from build123d import *

# Parameters (mm, degrees)
BOSS_EXTRUDE1_DEPTH            = 17
F_3_3_3_3_DIAMETER_HOLE1_D     = 3.3
F_3_3_3_3_DIAMETER_HOLE1_DEPTH = 25
F_3_3_3_3_DIAMETER_HOLE1_TIP   = 0.991420021


with BuildPart() as part:
    # Sketch1 → Boss-Extrude1 (new body)
    with BuildSketch(Plane.XY):
        with BuildLine():
            Line((-15, -23.643180835), (-15, -38))
            Line((-15, -38), (15, -38))
            Line((15, -38), (15, -23.643180835))
            ThreePointArc((15, -23.643180835), (0, 28), (-15, -23.643180835))
        make_face()
    extrude(amount=BOSS_EXTRUDE1_DEPTH)

    # Ø3.3 (3.3) Diameter Hole1
    with Locations(Plane.XY.offset(17)):
        with Locations((-23, 0), (23, 0)):
            Hole(F_3_3_3_3_DIAMETER_HOLE1_D / 2, depth=F_3_3_3_3_DIAMETER_HOLE1_DEPTH)
            with Locations((0, 0, -(F_3_3_3_3_DIAMETER_HOLE1_DEPTH + F_3_3_3_3_DIAMETER_HOLE1_TIP / 2))):  # 118° drill point
                Cone(0, F_3_3_3_3_DIAMETER_HOLE1_D / 2, F_3_3_3_3_DIAMETER_HOLE1_TIP, mode=Mode.SUBTRACT)


solid = part.part
Part model, mm, in its own coordinate system. A direction names the side the tool comes from. Coordinates: 2 decimals unless noted, no trailing zeros. Write each loop counter-clockwise with the first axis right and the second up, starting at its lowest first coordinate (ties: lowest second). Pieces come first, ordered by that corner, then holes. Notation, with made-up numbers: M 40,40.25 L 79,40.25 A23 cw 79,66.25 Z; hole C 12,70 d7. An arc over 180 degrees is marked long. Return JSON: item names as keys, results as strings.
1. Flat gauge pins, fed straight in: pin 1 Ø1 at (y, z) = (2.5, 12) entering from +X; pin 2 Ø4 at (y, z) = (17.5, 14.5) entering from -X; pin 3 Ø2 at (y, z) = (19.5, 8) entering from +X. Where does each tip first touch, or does it go through?
Determined:
{"pin 1": "x = 27.93", "pin 2": "x = -23.32", "pin 3": "x = 21.02"}
2. Saw through at D-D, the plane y = -28.5. Write the cut outline in (x, z).
Determined:
{"outline": "M -15,0 L 15,0 L 15,17 L -15,17 Z"}
3. Pull direction Y, two halves, no side cores. Call faces 4 (the face through (24.65, 0.07, 8.38)), 5 (the face through (0, -38, 8)), 6 (the face through (1.01, 27.98, 8.38)): pulls with the +Y half, pulls with the -Y half, needs draft (parallel to the pull), parting line crosses it, or undercut.
Determined:
{"face 4": "undercut", "face 5": "pulls with the -Y half", "face 6": "parting line crosses it"}
4. Saw through at C-C, the plane z = 2.25. Write the cut outline in (x, y).
Determined:
{"outline": "M -15,-38 L 15,-38 L 15,-23.64 A28 ccw long -15,-23.64 Z; hole C -23,0 d3.3; hole C 23,0 d3.3"}
5. 3-axis set-ups, long thin cutter, end or side, ignore diameter. For faces 1 (the face through (-15, -31, 8)), 2 (the face through (15, -31, 8)), 3 (the face through (0, -5, 17)): which of +Z, -Z, +X, -X, +Y, -Y reach the whole face in a straight line?
Determined:
{"face 1": "+Z, -Z, -X, -Y", "face 2": "+Z, -Z, +X, -Y", "face 3": "+Z, +X, -X, +Y, -Y"}
6. Saw through at B-B, the plane x = -23. Write the cut outline in (y, z).
Determined:
{"outline": "M -15.97,0 L -1.65,0 L -1.65,17 L -15.97,17 Z; M 1.65,0 L 15.97,0 L 15.97,17 L 1.65,17 Z"}
7. Probe L1, parallel to X at y = -27, z = 12.25; L2, parallel to Y at x = 23, z = 10; L3, parallel to Y at x = 24, z = 4. List the from-to ranges inside material, lowest first.
Determined:
{"L1": "-15 to 15", "L2": "-15.97 to -1.65, 1.65 to 15.97", "L3": "-14.42 to -1.31, 1.31 to 14.42"}
8. Saw through at A-A, the plane y = 0. Write the cut outline in (x, z).
Determined:
{"outline": "M -28,0 L -24.65,0 L -24.65,17 L -28,17 Z; M -21.35,0 L 21.35,0 L 21.35,17 L -21.35,17 Z; M 24.65,0 L 28,0 L 28,17 L 24.65,17 Z"}
